Design review of the part built by this model. Coordinates are the model's own, in mm. A direction names the side the tool comes from. Coordinates: 2 decimals unless noted, no trailing zeros. Loops run counter-clockwise (first coordinate to the right, second up) from the corner with the lowest first, then second, coordinate; pieces in that order, holes last.
Q1. Machinability: for faces 1 (the face through (51, 4, 14.475)), 2 (the face through (-52.5, 0, 15)), 3 (the face through (50.5, 0, 15)), which of the approach directions +Z, -Z, +X, -X, +Y, -Y give a long, thin tool a straight path to every point of the face, cutting with its end or side? Answer none if there is none.
Q2. Add section C-C on z = 11. Give the boundary of the cut face in (x, y), and give its area (3 significant figures).
Q3. Draft analysis for pull direction Y (two halves, no side actions). For faces 4 (the face through (-1, -30.5, 15)), 5 (the face through (-1, -32.5, 15)), 6 (the face through (-1, 30.5, 15)), 7 (the face through (52.5, 0, 15)), state which applies: released by +Y, released by -Y, zero draft, split by the parting line, or undercut.
Q4. Add section B-B on x = -13.5. Give the boundary of the cut face in (y, z).
Q5. Add section A-A on y = 3. Give the boundary of the cut face in (x, z), and give its area (3 significant figures).
Q6. Add section D-D on y = 26.5. Give the boundary of the cut face in (x, z), and give its area (3 significant figures).
Q7. Wall thickness on probe 1 along X at (y, z) = (-10, 21); probe 2 along Z at (x, y) = (51.25, -14.5); probe 3 along Y at (x, z) = (-39, 19.75): over which ranges is each line inside the solid? List them lowest first.
```python
from build123d import *

# Parameters (mm, degrees)
SKETCH004_W   = 65
SKETCH004_H   = 30
SKETCH004_R   = 2.5
SKETCH004_W_2 = 12
SKETCH004_H_2 = 4.5
PAD003_DEPTH  = 2
FILLET004_R   = 1
FILLET005_R   = 1
SKETCH002_W   = 105
SKETCH002_H   = 30
PAD001_DEPTH  = 2
FILLET002_R   = 1
FILLET003_R   = 1
SKETCH005_W   = 65
SKETCH005_H   = 30
PAD004_DEPTH  = 2
FILLET016_R   = 1
FILLET021_R   = 1
SKETCH003_W   = 105
SKETCH003_H   = 30
PAD002_DEPTH  = 2
FILLET009_R   = 1
FILLET017_R   = 1


with BuildPart() as body003:
    # Sketch004 → Pad003 (new body)
    with BuildSketch(Plane.YZ):
        with Locations((0, 15)):
            Rectangle(SKETCH004_W, SKETCH004_H)
        with Locations((-14.5, 11)):
            Circle(SKETCH004_R, mode=Mode.SUBTRACT)
        with Locations((3.989801, 12.224792)):
            Rectangle(SKETCH004_W_2, SKETCH004_H_2, mode=Mode.SUBTRACT)
    extrude(amount=PAD003_DEPTH)

    # Fillet004
    fillet004_edges = [body003.edges().sort_by_distance(p)[0] for p in [
        (2, 32.5, 15),
    ]]
    fillet(fillet004_edges, radius=FILLET004_R)

    # Fillet005
    fillet005_edges = [body003.edges().sort_by_distance(p)[0] for p in [
        (2, -32.5, 15),
    ]]
    fillet(fillet005_edges, radius=FILLET005_R)


with BuildPart() as body003_1:
    # Body003 placement: moved
    add(body003.part.moved(Location((50.5, 0, 0))))


with BuildPart() as body001:
    # Sketch002 → Pad001 (new body)
    with BuildSketch(Plane.XZ):
        with Locations((0, 15)):
            Rectangle(SKETCH002_W, SKETCH002_H)
    extrude(amount=PAD001_DEPTH)

    # Fillet002
    fillet002_edges = [body001.edges().sort_by_distance(p)[0] for p in [
        (-52.5, -2, 15),
    ]]
    fillet(fillet002_edges, radius=FILLET002_R)

    # Fillet003
    fillet003_edges = [body001.edges().sort_by_distance(p)[0] for p in [
        (52.5, -2, 15),
    ]]
    fillet(fillet003_edges, radius=FILLET003_R)


with BuildPart() as body001_1:
    # Body001 placement: moved
    add(body001.part.moved(Location((0, -30.5, 0))))


with BuildPart() as body004:
    # Sketch005 → Pad004 (new body)
    with BuildSketch(Plane.YZ):
        with Locations((0, 15)):
            Rectangle(SKETCH005_W, SKETCH005_H)
    extrude(amount=PAD004_DEPTH)

    # Fillet016
    fillet016_edges = [body004.edges().sort_by_distance(p)[0] for p in [
        (0, 32.5, 15),
    ]]
    fillet(fillet016_edges, radius=FILLET016_R)

    # Fillet021
    fillet021_edges = [body004.edges().sort_by_distance(p)[0] for p in [
        (0, -32.5, 15),
    ]]
    fillet(fillet021_edges, radius=FILLET021_R)


with BuildPart() as body004_1:
    # Body004 placement: moved
    add(body004.part.moved(Location((-52.5, 0, 0))))


with BuildPart() as body010:
    # Sketch003 → Pad002 (new body)
    with BuildSketch(Plane.XZ):
        with Locations((0, 15)):
            Rectangle(SKETCH003_W, SKETCH003_H)
    extrude(amount=PAD002_DEPTH)

    # Fillet009
    fillet009_edges = [body010.edges().sort_by_distance(p)[0] for p in [
        (52.5, 0, 15),
    ]]
    fillet(fillet009_edges, radius=FILLET009_R)

    # Fillet017
    fillet017_edges = [body010.edges().sort_by_distance(p)[0] for p in [
        (-52.5, 0, 15),
    ]]
    fillet(fillet017_edges, radius=FILLET017_R)


with BuildPart() as body010_1:
    # Body002 placement: moved
    add(body010.part.moved(Location((0, 32.5, 0))))

    # Fusion001: union Body003, Body001, Body004
    add(body003_1.part)
    add(body001_1.part)
    add(body004_1.part)


solid = body010_1.part
```
Entries:
1. face 1: +X
1. face 2: +Z, -Z, -X, +Y, -Y
1. face 3: +Z, -Z
2. outline: (-52.5, -31.5) arc R1 ccw to (-51.5, -32.5) - (51.5, -32.5) arc R1 ccw to (52.5, -31.5) - (52.5, -17) - (50.5, -17) - (50.5, -30.5) - (-50.5, -30.5) - (-50.5, 30.5) - (50.5, 30.5) - (50.5, 9.99) - (52.5, 9.99) - (52.5, 31.5) arc R1 ccw to (51.5, 32.5) - (-51.5, 32.5) arc R1 ccw to (-52.5, 31.5) - close; (50.5, -12) - (52.5, -12) - (52.5, -2.01) - (50.5, -2.01) - close
2. area: 629 mm2
3. face 4: undercut
3. face 5: released by -Y
3. face 6: undercut
3. face 7: zero draft
4. outline: (-32.5, 0) - (-30.5, 0) - (-30.5, 30) - (-32.5, 30) - close; (30.5, 0) - (32.5, 0) - (32.5, 30) - (30.5, 30) - close
5. outline: (-52.5, 0) - (-50.5, 0) - (-50.5, 30) - (-52.5, 30) - close; (50.5, 0) - (52.5, 0) - (52.5, 9.97) - (50.5, 9.97) - close; (50.5, 14.47) - (52.5, 14.47) - (52.5, 30) - (50.5, 30) - close
5. area: 111 mm2
6. outline: (-52.5, 0) - (-50.5, 0) - (-50.5, 30) - (-52.5, 30) - close; (50.5, 0) - (52.5, 0) - (52.5, 30) - (50.5, 30) - close
6. area: 120 mm2
7. probe 1: x = -52.5 to -50.5, 50.5 to 52.5
7. probe 2: z = 0 to 8.5, 13.5 to 30
7. probe 3: y = -32.5 to -30.5, 30.5 to 32.5
